Verification items for the finished model (mm, model axes). Face numbers are marked on the shaded views. A direction names the side the tool comes from. Coordinates: 2 decimals unless noted, no trailing zeros. Order: outer loops, then holes, each group sorted by start corner. A loop starts at its lowest first (then second) coordinate and runs counter-clockwise, first axis right, second up. Notation, with made-up numbers: M 1,51 L 36,51 A28 cw 36,81 Z; hole C -16.75,-8 d4. An arc over 180 degrees is marked long. Return JSON: item names as keys, results as strings. Group by question number.
Q1. Access from +Z, -Z, +X, -X, +Y, -Y to the whole of each face (thin tool, end or side, straight path). Record for the marked faces 1, 2, 3 and 4.
Q2. Section check B-B, the plane z = -3.5. Enter the section's corners in (x, y).
Q3. Section check C-C, the plane z = -17.75. Enter the section's corners in (x, y), then the cut area to 3 significant figures.
Q4. Section check A-A, the plane x = -12.5. Enter the section's corners in (y, z), then the cut area to 3 significant figures.
Q5. Go/stop test with flat-tipped pins: pin 1 Ø1.5 at (y, z) = (-0.5, -13) entering from -X; pin 2 Ø2.5 at (y, z) = (-5, -9) entering from +X; pin 3 Ø4 at (y, z) = (3, -15.5) entering from +X. Record where each tip stops, or that it passes through.
Q6. Thickness scan on probe 1 along Y at (x, z) = (-33.6, -8.55); probe 2 along Z at (x, y) = (5.5, -3); probe 3 along Y at (x, z) = (-4, -14.25). Record the ranges inside material, lowest first.
from build123d import *

# Parameters (mm, degrees)
BOSS_EXTRUDE1_DEPTH     = 10.3
BOSS_EXTRUDE2_DEPTH     = 20.5
CUT_EXTRUDE1_DEPTH      = 40.4825911
CUT_EXTRUDE1_DEPTH_BACK = 40.4825911
SKETCH3_R               = 1.65
BOSS_EXTRUDE3_DEPTH     = 3


with BuildPart() as part:
    # Sketch1 → Boss-Extrude1 (new body)
    with BuildSketch(Plane.XY):
        Polygon((-33.25, -5.75), (33.25, -5.75), (26.610471904, 5.75), (-26.610471904, 5.75), align=None)
    extrude(amount=-BOSS_EXTRUDE1_DEPTH)

    # Sketch1<5> → Boss-Extrude2 (add)
    with BuildSketch(Plane.XY):
        Polygon((-28.486860279, 2.5), (-31.373611625, -2.5), (31.373611625, -2.5), (28.486860279, 2.5), align=None)
    extrude(amount=-BOSS_EXTRUDE2_DEPTH)

    # Sketch2 → Cut-Extrude1 (cut, two sides: drawn at the far end of the back side and taken through both)
    with BuildSketch(Plane(origin=(0, 0, 0), x_dir=(0, 0, -1), z_dir=(1, 0, 0)).offset(-CUT_EXTRUDE1_DEPTH_BACK)):
        Polygon((20.5, -2.5), (14.3, 2.5), (20.5, 2.5), align=None)
    extrude(amount=CUT_EXTRUDE1_DEPTH + CUT_EXTRUDE1_DEPTH_BACK, mode=Mode.SUBTRACT)

    # Sketch3 → Boss-Extrude3 (add)
    with BuildSketch(Plane(origin=(0, 0, -10.3), x_dir=(-1, 0, 0), z_dir=(0, 0, -1))):
        with BuildLine():
            Line((-33.25, -5.75), (-34.6, -5.75))
            Line((-34.6, -5.75), (-34.6, -2.892116168))
            ThreePointArc((-34.6, -2.892116168), (-37.064101615, 2.980867179), (-30.745898034, 3.783384256))
            Line((-30.745898034, 3.783384256), (-29.610471904, 5.75))
            Line((-29.610471904, 5.75), (-26.610471904, 5.75))
            Line((-26.610471904, 5.75), (-33.25, -5.75))
        make_face()
        with Locations((-33.6, 0.980867179)):
            Circle(SKETCH3_R, mode=Mode.SUBTRACT)
    boss_extrude3 = extrude(amount=-BOSS_EXTRUDE3_DEPTH)

    # Mirror1: Boss-Extrude3 across plane
    add(boss_extrude3.mirror(Plane(origin=(0, 0, 0), x_dir=(0, 0, 1), z_dir=(1, 0, 0))))


solid = part.part
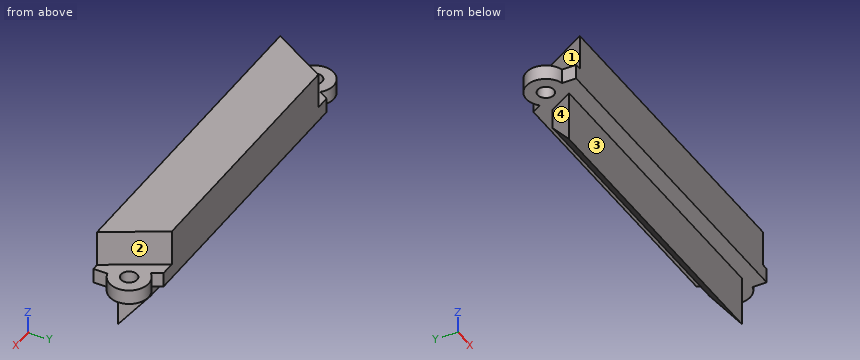
Numbers:
{
 "1": {"face 1": "+Z, -X, +Y", "face 2": "+Z, +X, +Y", "face 3": "-Z, +X, -X, -Y", "face 4": "-Z, -X, +Y"},
 "2": {"outline": "M -33.25,-5.75 L 33.25,-5.75 L 26.61,5.75 L -26.61,5.75 Z"},
 "3": {"outline": "M -31.37,-2.5 L 31.37,-2.5 L 30.09,-0.28 L -30.09,-0.28 Z", "area": "136 mm2"},
 "4": {"outline": "M -5.75,-10.3 L -2.5,-10.3 L -2.5,-20.5 L 2.5,-14.3 L 2.5,-10.3 L 5.75,-10.3 L 5.75,0 L -5.75,0 Z", "area": "154 mm2"},
 "5": {"pin 1": "stops at x = -30.65", "pin 2": "stops at x = 34.6", "pin 3": "stops at x = 29.35"},
 "6": {"probe 1": "y = -5.75 to -0.67, 2.63 to 4.98", "probe 2": "z = -10.3 to 0", "probe 3": "y = -2.5 to 2.5"}
}
